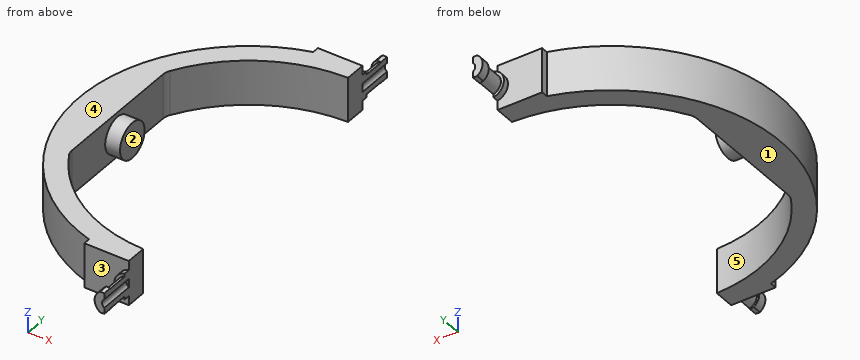
```python
from build123d import *

# Parameters (mm, degrees)
F1_DEPTH  = 15
F2_R      = 6
F3_DEPTH  = 5
F4_R      = 5
F6_DEPTH  = 2
F8_DEPTH  = 7
F10_DEPTH = 3
F11_DEPTH = 25
F13_W     = 146.8421146274
F13_H     = 28.1250011176
F14_DEPTH = 1
F15_W     = 11.3657170441
F15_H     = 11.5304403007
F15_W_2   = 13.3423628286
F15_H_2   = 13.0129233003
F16_DEPTH = 4
F17_W     = 19.5150814822
F17_H     = 12.7272193491
F17_W_2   = 18.9494257321
F17_H_2   = 10.7474377315
F18_DEPTH = 4


with BuildPart() as f1:
    # F0 (on Top) → F1 (new body)
    with BuildSketch(Plane.XY):
        with BuildLine():
            ThreePointArc((-44.16, 23.4498272915), (-25.7634298515, 42.8514373421), (0, 50))
            Line((0, 50), (0, 57))
            Line((0, 57), (-15.9976914198, 57))
            Line((-15.9976914198, 57), (-15.9976914198, 54.7089925811))
            ThreePointArc((-15.9976914198, 54.7089925811), (-57, 0), (-15.9976914198, -54.7089925811))
            Line((-15.9976914198, -54.7089925811), (-15.9976914198, -57))
            Line((-15.9976914198, -57), (0, -57))
            Line((0, -57), (0, -50))
            ThreePointArc((0, -50), (-25.7634298515, -42.8514373421), (-44.16, -23.4498272915))
            Line((-44.16, -23.4498272915), (-44.16, 23.4498272915))
        make_face()
    extrude(amount=F1_DEPTH)

    # F2 (on face) → F3 (join)
    with BuildSketch(Plane.YZ.offset(-44.16)):
        with Locations((0, 7.5)):
            Circle(F2_R)
    extrude(amount=F3_DEPTH)

    # F4
    f4_edges = [f1.edges().sort_by_distance(p)[0] for p in [
        (-44.16, 23.449827, 7.5),
        (-44.16, -23.449827, 7.5),
    ]]
    fillet(f4_edges, radius=F4_R)

    # F5 (on face) → F6 (join)
    with BuildSketch(Plane.XZ.offset(57)):
        with BuildLine():
            Line((0, 9.25), (0, 12))
            ThreePointArc((0, 12), (-4.5, 7.5), (0, 3))
            Line((0, 3), (0, 5.75))
            ThreePointArc((0, 5.75), (-1.75, 7.5), (0, 9.25))
        make_face()
    extrude(amount=F6_DEPTH)

    # F7 (on face) → F8 (join)
    with BuildSketch(Plane.XZ.offset(59)):
        with BuildLine():
            Line((0, 9.25), (0, 11))
            ThreePointArc((0, 11), (-3.5, 7.5), (0, 4))
            Line((0, 4), (0, 5.75))
            ThreePointArc((0, 5.75), (-1.75, 7.5), (0, 9.25))
        make_face()
    extrude(amount=F8_DEPTH)

    # F9 (on face) → F10 (join)
    with BuildSketch(Plane.XZ.offset(66)):
        with BuildLine():
            Line((0, 3.25), (0, 11.75))
            ThreePointArc((0, 11.75), (-4.25, 7.5), (0, 3.25))
        make_face()
    extrude(amount=F10_DEPTH)

    # F11 (cut): a face of the model
    f11_faces = [f1.faces().sort_by_distance(p)[0] for p in [
        (-0.7427230678, -66, 7.5),
    ]]
    extrude(f11_faces, amount=-F11_DEPTH, mode=Mode.SUBTRACT)

    # F12: F1 across plane


with BuildPart() as f1_1:
    add(f1.part)
    add(f1.part.mirror(Plane.XZ))

    # F13 (on Right) → F14 (cut)
    with BuildSketch(Plane.YZ):
        with Locations((0.2960525453, 7.5493426993)):
            Rectangle(F13_W, F13_H)
    extrude(amount=-F14_DEPTH, mode=Mode.SUBTRACT)

    # F15 (on Top) → F16 (cut)
    with BuildSketch(Plane.XY):
        with Locations((-1.9552764716, -64.7652201504)):
            Rectangle(F15_W, F15_H)
        with Locations((-2.1199961193, 65.5064616501)):
            Rectangle(F15_W_2, F15_H_2)
    extrude(amount=F16_DEPTH, mode=Mode.SUBTRACT)

    # F17 (on face) → F18 (cut)
    with BuildSketch(Plane.XY.offset(15)):
        with Locations((-4.4578294758, 65.3636096745)):
            Rectangle(F17_W, F17_H)
        with Locations((-2.7608656596, -64.3737188657)):
            Rectangle(F17_W_2, F17_H_2)
    extrude(amount=-F18_DEPTH, mode=Mode.SUBTRACT)


solid = f1_1.part
```
Source: CAD feature listing. Evaluate the final solid. Frame: model axes, mm. Face numbers are marked on the shaded views. A direction names the side the tool comes from. Give positions to 0.01 mm unless a question says otherwise; leave off trailing zeros. Loops run counter-clockwise (first coordinate to the right, second up) from the corner with the lowest first, then second, coordinate; pieces in that order, holes last. Notation, with made-up numbers: (11, 46) -> (32, 46) arc R30 ccw to (32, 74) -> close; hole circle Ø6 at (60, 16.25). An arc over 180 degrees is marked (long way). Put each result on its own line as item: value. Start each with the question number.
1) Contact query for flat-ended pins moving along their axis: P1, Ø5, axis at x = -14.5, z = 4, coming from the -Y side; P2, Ø1.6, axis at x = -1.5, y = 67, coming from the +Z side; P3, Ø0.7, axis at y = 56, z = 10.5, coming from the -X side. Output: stop coordinate, or through.
2) Draft query along Y for the marked faces 1, 2 and 3. Return one class per face: released by +Y, released by -Y, zero draft, split by the parting line, or undercut.
3) Material intervals for probe 1 along Y at (x, z) = (-7, 7.75); probe 2 along Y at (x, z) = (-26, 4); probe 3 along X at (y, z) = (34, 2), sorted ascending.
4) Cut plane A-A (x = -19.5). Return loops of the section in (y, z), then the cut area to 3 significant figures.
5) Reachability of the marked faces 4 and 5 from +Z, -Z, +X, -X, +Y, -Y: full face, straight path, thin tool, end or side. Return the list, or none.
6) Cut plane C-C (y = 0). Return loops of the section in (x, z), then the cut area to 3 significant figures.
7) Cut plane D-D (x = -8). Return loops of the section in (y, z).
Results are:
1. P1: stops at y = -57
1. P2: stops at z = 11
1. P3: stops at x = -16
2. face 1: zero draft
2. face 2: undercut
2. face 3: released by -Y
3. probe 1: y = -57 to -49.51, 49.51 to 57
3. probe 2: y = -50.72 to -42.71, 42.71 to 50.72
3. probe 3: x = -45.75 to -36.66
4. outline: (-53.56, 0) -> (-46.04, 0) -> (-46.04, 15) -> (-53.56, 15) -> close; (46.04, 0) -> (53.56, 0) -> (53.56, 15) -> (46.04, 15) -> close
4. area: 226 mm2
5. face 4: +Z, +X, -X, +Y, -Y
5. face 5: +Z, -Z, +X
6. outline: (-57, 0) -> (-44.16, 0) -> (-44.16, 1.5) -> (-39.16, 1.5) -> (-39.16, 13.5) -> (-44.16, 13.5) -> (-44.16, 15) -> (-57, 15) -> close
6. area: 253 mm2
7. outline: (-57, 0) -> (-49.36, 0) -> (-49.36, 15) -> (-57, 15) -> close; (49.36, 0) -> (57, 0) -> (57, 15) -> (49.36, 15) -> close
